from build123d import *

# Parameters (mm, degrees)
F0_W     = 31.8
F0_H     = 15.8
F1_DEPTH = 9.8
F2_R     = 2.4
F3_DEPTH = 1.8
F4_W     = 30.6
F4_H     = 14.6
F5_DEPTH = 6.6
F6_R     = 1.3
F7_DEPTH = 1.7
F8_R     = 3.25
F8_R_2   = 2.3
F9_DEPTH = 6.6


with BuildPart() as f1:
    # F0 (on Top) → F1 (new body)
    with BuildSketch(Plane.XY):
        with Locations((15.9, 7.9)):
            Rectangle(F0_W, F0_H)
    extrude(amount=F1_DEPTH)

    # F2 (on face) → F3 (join)
    with BuildSketch(Plane.XY.offset(9.8)):
        with Locations((3.9, 12.384264)):
            Circle(F2_R)
        with Locations((28.124928, 4.057131)):
            Circle(F2_R)
        with Locations((27.9, 12.384264)):
            Circle(F2_R)
        with Locations((19.9, 12.384264)):
            Circle(F2_R)
        with Locations((20.124928, 4.057131)):
            Circle(F2_R)
        with Locations((11.9, 12.384264)):
            Circle(F2_R)
        with Locations((12.124928, 4.057131)):
            Circle(F2_R)
        with Locations((4.124928, 4.057131)):
            Circle(F2_R)
    extrude(amount=F3_DEPTH)

    # F4 (on face) → F5 (cut)
    with BuildSketch(Plane(origin=(0, 0, 0), x_dir=(1, 0, 0), z_dir=(0, 0, -1))):
        with Locations((15.9, -7.9)):
            Rectangle(F4_W, F4_H)
    extrude(amount=-F5_DEPTH, mode=Mode.SUBTRACT)

    # F6 (on face) → F7 (cut)
    with BuildSketch(Plane(origin=(0, 0, 6.6), x_dir=(1, 0, 0), z_dir=(0, 0, -1))):
        with Locations((3.614632, -3.203599)):
            Circle(F6_R)
        with Locations((11.614632, -3.203599)):
            Circle(F6_R)
        with Locations((19.614632, -3.203599)):
            Circle(F6_R)
        with Locations((27.614632, -3.203599)):
            Circle(F6_R)
        with Locations((27.614632, -11.203599)):
            Circle(F6_R)
        with Locations((19.614632, -11.203599)):
            Circle(F6_R)
        with Locations((11.614632, -11.203599)):
            Circle(F6_R)
        with Locations((3.614632, -11.203599)):
            Circle(F6_R)
    extrude(amount=-F7_DEPTH, mode=Mode.SUBTRACT)

    # F8 (on face) → F9 (join)
    with BuildSketch(Plane(origin=(0, 0, 6.6), x_dir=(1, 0, 0), z_dir=(0, 0, -1))):
        with Locations((7.414678, -7.084377)):
            Circle(F8_R)
        with Locations((7.414678, -7.084377)):
            Circle(F8_R_2, mode=Mode.SUBTRACT)
        with Locations((15.914678, -7.084377)):
            Circle(F8_R)
        with Locations((15.914678, -7.084377)):
            Circle(F8_R_2, mode=Mode.SUBTRACT)
        with Locations((24.414678, -7.084377)):
            Circle(F8_R)
        with Locations((24.414678, -7.084377)):
            Circle(F8_R_2, mode=Mode.SUBTRACT)
    extrude(amount=F9_DEPTH)


solid = f1.part
For this review, take the finished solid that the model builds, in its own axes (mm). A direction names the side the tool comes from. Round coordinates to 2 decimals unless told otherwise and drop trailing zeros. Loops run counter-clockwise (first coordinate to the right, second up) from the corner with the lowest first, then second, coordinate; pieces in that order, holes last. Notation, with made-up numbers: (34.5, 66) - (64.5, 66) arc R26 ccw to (64.5, 101) - close; hole circle Ø7 at (27.5, 59.5). An arc over 180 degrees is marked (long way). Put each result on its own line as item: value. Start each with the question number.
1. Consider section B-B on x = 3. State the section outline as (y, z) points, plus the area to 3 significant figures.
2. Insertion check: P1, Ø3, axis at x = 3.5, y = 3, coming from the -Z side; P2, Ø0.8, axis at x = 12, y = 10.5, coming from the -Z side. Each pin has a flat end and moves straight along its axis. Give the tip position at first contact, or say it passes through.
3. Consider section A-A on z = 4.5. State the section outline as (x, y) points, plus the area to 3 significant figures.
4. Mouldability with a two-part tool opening along Y and no side actions: class faces 1 (the cylindrical face through (14.342, 3.138, 10.687)), 2 (the flat face through (12, 4, 11.6)) as +Y half, -Y half, draft (parallel to the pull), parting line (faces both ways), or undercut.
5. Consider section D-D on x = 17. State the section outline as (y, z) points, plus the area to 4 significant figures.
6. For faces 3 (the cylindrical face through (5.232, 1.928, 10.687)), 4 (the flat face through (11.1, 0.3, 0)), 5 (the cylindrical face through (12.816, 3.702, 7.438)), list the 3-axis set-ups (+Z, -Z, +X, -X, +Y, -Y) from which the entire face can be reached by the end or side of a thin tool; tool diameter is ignored.
7. For probe 1 along Y at (x, z) = (7.5, 5.75); probe 2 along X at (y, z) = (13.75, 5.5); probe 3 along X at (y, z) = (4, 8), list the stretches that pass through material, from the lowest coordinate up. Write a range as [from, to].
Result sheet:
1. outline: (0, 0) - (0.6, 0) - (0.6, 6.6) - (2.06, 6.6) - (2.06, 8.3) - (4.35, 8.3) - (4.35, 6.6) - (10.06, 6.6) - (10.06, 8.3) - (12.35, 8.3) - (12.35, 6.6) - (15.2, 6.6) - (15.2, 0) - (15.8, 0) - (15.8, 9.8) - (14.61, 9.8) - (14.61, 11.6) - (10.16, 11.6) - (10.16, 9.8) - (6.18, 9.8) - (6.18, 11.6) - (1.94, 11.6) - (1.94, 9.8) - (0, 9.8) - close
1. area: 66.3 mm^2
2. P1: z = 6.6
2. P2: z = 8.3
3. outline: (0, 0) - (31.8, 0) - (31.8, 15.8) - (0, 15.8) - close; circle Ø6.5 at (7.41, 7.08); circle Ø6.5 at (15.91, 7.08); circle Ø6.5 at (24.41, 7.08); hole (0.6, 0.6) - (31.2, 0.6) - (31.2, 15.2) - (0.6, 15.2) - close; hole circle Ø4.6 at (7.41, 7.08); hole circle Ø4.6 at (15.91, 7.08); hole circle Ø4.6 at (24.41, 7.08)
3. area: 105 mm^2
4. face 1: undercut
4. face 2: draft
5. outline: (0, 0) - (0.6, 0) - (0.6, 6.6) - (4.02, 6.6) - (4.02, 0) - (5.06, 0) - (5.06, 6.6) - (9.11, 6.6) - (9.11, 0) - (10.15, 0) - (10.15, 6.6) - (15.2, 6.6) - (15.2, 0) - (15.8, 0) - (15.8, 9.8) - (0, 9.8) - close
5. area: 72.15 mm^2
6. face 3: +Z
6. face 4: -Z, +X, -X, +Y, -Y
6. face 5: -Z
7. probe 1: [0, 0.6], [3.84, 4.79], [9.38, 10.33], [15.2, 15.8]
7. probe 2: [0, 0.6], [31.2, 31.8]
7. probe 3: [0, 2.59], [4.64, 10.59], [12.64, 18.59], [20.64, 26.59], [28.64, 31.8]
